from build123d import *

# Parameters (mm, degrees)
F0_W     = 76.734344
F0_H     = 49.875418
F1_DEPTH = 76.2
F2_R     = 5.879825
F3_DEPTH = 50.8


with BuildPart() as f1:
    # F0 (on Front) → F1 (new body)
    with BuildSketch(Plane.XZ):
        with Locations((-17.182841, -4.724878)):
            Rectangle(F0_W, F0_H)
    extrude(amount=-F1_DEPTH)

    # F2 (on face) → F3 (cut)
    with BuildSketch(Plane.XY.offset(20.212831)):
        with Locations((-47.513243, 12.172232)):
            Circle(F2_R)
    extrude(amount=-F3_DEPTH, mode=Mode.SUBTRACT)


solid = f1.part
Input: part model. Units: mm. Frame: model coordinates. Coordinates: 2 decimals unless noted, no trailing zeros. Write each loop counter-clockwise with the first axis right and the second up, starting at its lowest first coordinate (ties: lowest second). Pieces come first, ordered by that corner, then holes. Notation, with made-up numbers: M 22.5,6 L 38.5,6 A24 cw 38.5,41 Z; hole C 26,-36.75 d2. An arc over 180 degrees is marked long. Answer as a JSON object with one key per item and string values. Group by question number.
(1) Section A-A on y = 17. Output: boundary loops of the cut face in (x, z), plus the area to 3 significant figures.
(2) Mould query, pull axis Y, two halves, no side actions, for faces 1 (the face through (-44.35, 17.13, -4.38)), 2 (the face through (21.184, 38, -5)), 3 (the face through (-18, 0, -4)). Classes: pulls with the +Y half, pulls with the -Y half, needs draft (parallel to the pull), parting line crosses it, or undercut.
(3) Section B-B on z = 17. Output: boundary loops of the cut face in (x, y), plus the area to 3 significant figures.
(4) Ray query, line 1 along Y through (x, z) = (-43.5, -10) (3 decimals). Return the intervals inside material, ascending. Write a range as [from, to].
Result set:
{
 "1": {"outline": "M -55.55,-29.66 L -50.87,-29.66 L -50.87,20.21 L -55.55,20.21 Z; M -44.16,-29.66 L 21.18,-29.66 L 21.18,20.21 L -44.16,20.21 Z", "area": "3,490 mm2"},
 "2": {"face 1": "undercut", "face 2": "needs draft", "face 3": "pulls with the -Y half"},
 "3": {"outline": "M -55.55,0 L 21.18,0 L 21.18,76.2 L -55.55,76.2 Z; hole C -47.51,12.17 d11.76", "area": "5,740 mm2"},
 "4": {"line 1": "y = [0, 7.875], [16.469, 76.2]"}
}
